Here's the drawing with two shaded views (mm, measured from the low corner). I have some questions. Give positions to 0.01 mm unless a question says otherwise; leave off trailing zeros. Write each loop counter-clockwise with the first axis right and the second up, starting at its lowest first coordinate (ties: lowest second). Pieces come first, ordered by that corner, then holes. Notation, with made-up numbers: M 50,-39 L 103,-39 A20 ccw 103,-14 Z; hole C 63,66.25 d2. An arc over 180 degrees is marked long. Use one line per item in the form item = value.
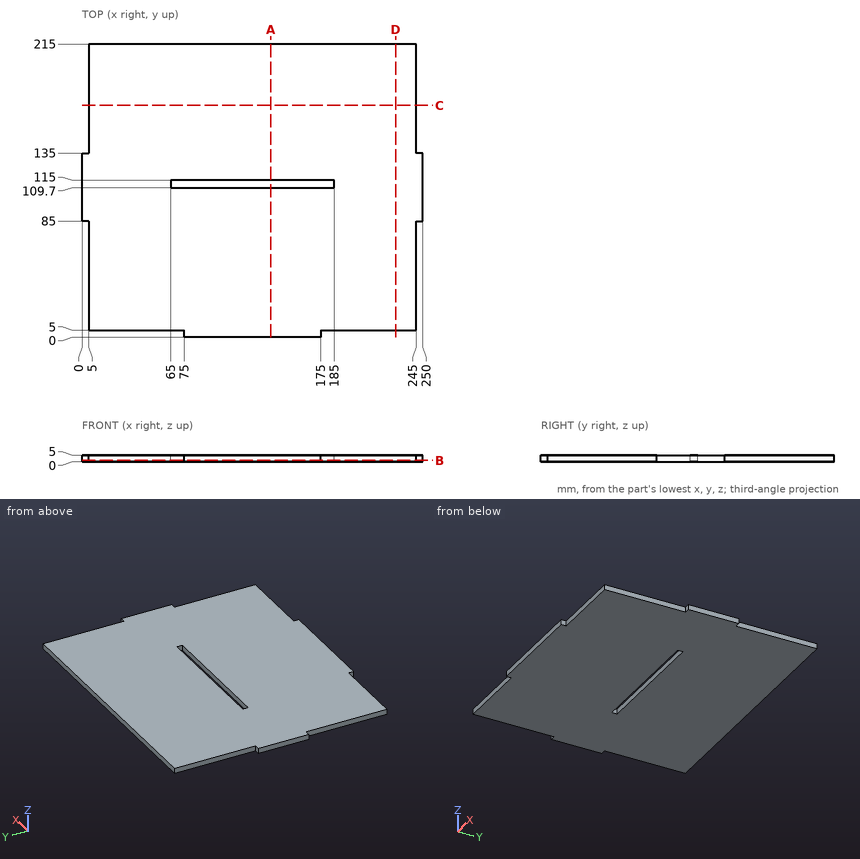
1) I want a section at D-D, the plane x = 230. Please give me the cut outline in (y, z).
Checked values:
outline = M 5,0 L 215,0 L 215,5 L 5,5 Z
2) If I drill on L1, parallel to Y at x = 124.5, z = 1.85; L2, parallel to Y at x = 18, z = 4.1; L3, parallel to X at y = 176.5, z = 3.4, over which ranges is the centre line in solid material (lowest first)?
Checked values:
L1 = 0 to 109.7, 115 to 215
L2 = 5 to 215
L3 = 5 to 245
3) I want a section at B-B, the plane z = 1.1. Please give me the cut outline in (x, y), plus the area to 3 significant figures.
Checked values:
outline = M 0,85 L 5,85 L 5,5 L 75,5 L 75,0 L 175,0 L 175,5 L 245,5 L 245,85 L 250,85 L 250,135 L 245,135 L 245,215 L 5,215 L 5,135 L 0,135 Z; hole M 65,109.7 L 185,109.7 L 185,115 L 65,115 Z
area = 50,800 mm2
4) For pin 1 Ø1.5 at (y, z) = (53, 1.5) entering from -X; pin 2 Ø2 at (x, z) = (66, 1) entering from -Y; pin 3 Ø2.5 at (x, z) = (1.5, 2.5) entering from +Y, each with a flat end and sliding along its axis, tell me the tip position at first contact or that it passes through.
Checked values:
pin_1 = 5
pin_2 = 5
pin_3 = 135
5) I want a section at A-A, the plane x = 138.5. Please give me the cut outline in (y, z), plus the area to 3 significant figures.
Checked values:
outline = M 0,0 L 109.7,0 L 109.7,5 L 0,5 Z; M 115,0 L 215,0 L 215,5 L 115,5 Z
area = 1,050 mm2
6) I want a section at C-C, the plane y = 170. Please give me the cut outline in (x, z), plus the area to 3 significant figures.
Checked values:
outline = M 5,0 L 245,0 L 245,5 L 5,5 Z
area = 1,200 mm2
